Verification items for the finished model (mm, model axes). A direction names the side the tool comes from. Coordinates: 2 decimals unless noted, no trailing zeros. Order: outer loops, then holes, each group sorted by start corner. A loop starts at its lowest first (then second) coordinate and runs counter-clockwise, first axis right, second up.
Q1. Depth check by flat-ended pin: P1, Ø3, axis at x = 0, z = 17.5, coming from the +Y side; P2, Ø5, axis at y = 3.5, z = 3.5, coming from the +X side; P3, Ø1.5, axis at y = 3.5, z = 10.5, coming from the -X side. Enter the tip coordinate at first touch or a pass-through.
Q2. Cross-section at C-C, the plane z = 6.25. Record the boundary of the cut face in (x, y), and give its area (3 significant figures).
Q3. Set-up check for faces 4 (the cylindrical face through (-1.617, -0.67, 4.93)), 5 (the flat face through (0, -2, 10)): record each of +Z, -Z, +X, -X, +Y, -Y from which the full face is reachable in a straight line by a thin tool's end or side.
Q4. Draft check along X on faces 1 (the cylindrical face through (-7.493, 0.33, 7.828)), 2 (the flat face through (0, 2, 0)), 3 (the cylindrical face through (-1.19, -5.37, 15.07)). Enter one of: pulls with the +X half, pulls with the -X half, needs draft (parallel to the pull), parting line crosses it, or undercut.
Q5. Cross-section at A-A, the plane x = 0. Record the boundary of the cut face in (y, z), and give its area (3 significant figures).
Q6. Thickness scan on line 1 (Y direction, x = 0, z = 15.5); line 2 (Y direction, x = 0, z = 6.25); line 3 (Z direction, x = -3.75, y = -1.5). Record the ranges inside material, lowest first.
from build123d import *

# Parameters (mm, degrees)
SKETCH1_R           = 7.5
BOSS_EXTRUDE1_DEPTH = 20
SKETCH2_R           = 5.5
CUT_EXTRUDE1_DEPTH  = 10
CHAMFER1_SIZE       = 1.5
CHAMFER1_SIZE2      = 4.121216129
SKETCH3_R           = 1.75
CUT_EXTRUDE2_DEPTH  = 23.638462845


with BuildPart() as part:
    # Sketch1 → Boss-Extrude1 (new body)
    with BuildSketch(Plane.XY):
        Circle(SKETCH1_R)
    extrude(amount=BOSS_EXTRUDE1_DEPTH)

    # Sketch2 → Cut-Extrude1 (cut)
    with BuildSketch(Plane.XY.offset(20)):
        Circle(SKETCH2_R)
    extrude(amount=-CUT_EXTRUDE1_DEPTH, mode=Mode.SUBTRACT)

    # Chamfer1
    chamfer1_edges = [part.edges().sort_by_distance(p)[0] for p in [
        (-7.5, 0, 20),
    ]]
    chamfer1_side = [part.faces().sort_by_distance(p)[0] for p in [
        (-7.287867966, 0, 20),
    ]]
    chamfer(chamfer1_edges, length=CHAMFER1_SIZE, length2=CHAMFER1_SIZE2, reference=chamfer1_side[0])

    # Sketch3 → Cut-Extrude2 (cut, through all)
    with BuildSketch(Plane(origin=(0, 0, 0), x_dir=(-1, 0, 0), z_dir=(0, 0, -1))):
        Circle(SKETCH3_R)
    extrude(amount=-CUT_EXTRUDE2_DEPTH, mode=Mode.SUBTRACT)


solid = part.part
Check values:
1. P1: stops at y = 7.46
1. P2: stops at x = 7.43
1. P3: stops at x = -6.98
2. outline: circle Ø15 at (0, 0); hole circle Ø3.5 at (0, 0)
2. area: 167 mm2
3. face 4: +Z, -Z
3. face 5: +Z
4. face 1: parting line crosses it
4. face 2: needs draft
4. face 3: undercut
5. outline: (-7.5, 0) - (-1.75, 0) - (-1.75, 10) - (-5.5, 10) - (-5.5, 20) - (-6, 20) - (-7.5, 15.88) - close; (1.75, 0) - (7.5, 0) - (7.5, 15.88) - (6, 20) - (5.5, 20) - (5.5, 10) - (1.75, 10) - close
5. area: 149 mm2
6. line 1: y = -7.5 to -5.5, 5.5 to 7.5
6. line 2: y = -7.5 to -1.75, 1.75 to 7.5
6. line 3: z = 0 to 10
